The figure shows three views and two pictorial views of one solid part (mm, origin at its lowest corner). Answer the questions. A direction names the side the tool comes from. Give positions to 0.01 mm unless a question says otherwise; leave off trailing zeros. Order: outer loops, then holes, each group sorted by start corner. A loop starts at its lowest first (then second) coordinate and runs counter-clockwise, first axis right, second up. Notation, with made-up numbers: (59, 1.5) - (76, 1.5) arc R12 ccw to (76, 7.5) - close; hole circle Ø6 at (26.5, -32.5). An arc over 180 degrees is marked (long way). Answer as CSV lines item,"result". Start each with the question number.
1. Which of the six approach directions +Z, -Z, +X, -X, +Y, -Y give full straight-line access (tool end or side, diameter ignored) to the marked faces 5 and 6?
2. Flat-ended cylindrical pins translate along their axes: pin 1 (1 mm diameter, centred on x = 2.5, z = 7.5, fed in from -Y); pin 2 (4 mm diameter, centred on x = 5.5, y = 6, fed in from -Z); pin 3 (2 mm diameter, centred on y = 6.5, z = 8, fed in from -X) (1 decimal). Find the tip coordinate at first contact, or state that the pin passes through.
3. Determine the mould class of the marked faces 1, 2, 3 and 4 for opening direction X: +X half, -X half, draft (parallel to the pull), parting line (faces both ways), or undercut.
4. Section A-A on y = 10.25 is taken. Give the vertices of the cut face in (x, z).
5. Section B-B on x = 5 is taken. Give the vertices of the cut face in (y, z).
6. Consider line 1 along Y through (x, z) = (6.5, 3); line 2 along Y through (x, z) = (2, 2.25); line 3 along Z through (x, y) = (4, 5.25). Determine where each line is inside the solid, lowest interval first. Write a range as [from, to].
7. Section C-C on z = 4 is taken. Give the vertices of the cut face in (x, y).
8. Section D-D on y = 3.5 is taken. Give the vertices of the cut face in (x, z).
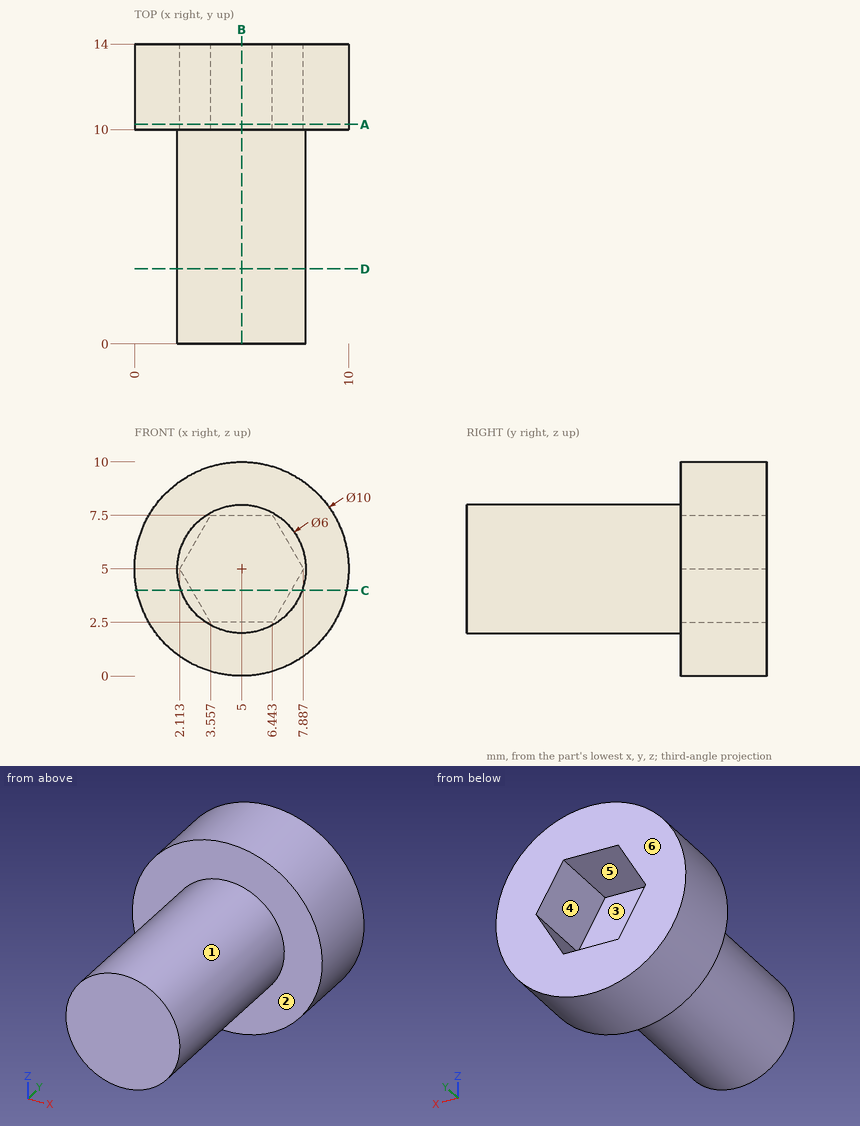
Checks:
1,face 5,"+Y"
1,face 6,"+Z, -Z, +X, -X, +Y"
2,pin 1,"stops at y = 10"
2,pin 2,"stops at z = 2"
2,pin 3,"stops at x = 2.8"
3,face 1,"parting line"
3,face 2,"draft"
3,face 3,"undercut"
3,face 4,"undercut"
4,outline,"circle Ø10 at (5, 5); hole (2.11, 5) - (3.56, 2.5) - (6.44, 2.5) - (7.89, 5) - (6.44, 7.5) - (3.56, 7.5) - close"
5,outline,"(0, 2) - (10, 2) - (10, 0) - (14, 0) - (14, 2.5) - (10, 2.5) - (10, 7.5) - (14, 7.5) - (14, 10) - (10, 10) - (10, 8) - (0, 8) - close"
6,line 1,"y = [0, 10]"
6,line 2,"y = [10, 14]"
6,line 3,"z = [2.17, 7.83]"
7,outline,"(0.1, 10) - (2.17, 10) - (2.17, 0) - (7.83, 0) - (7.83, 10) - (9.9, 10) - (9.9, 14) - (7.31, 14) - (7.31, 10) - (2.69, 10) - (2.69, 14) - (0.1, 14) - close"
8,outline,"circle Ø6 at (5, 5)"
